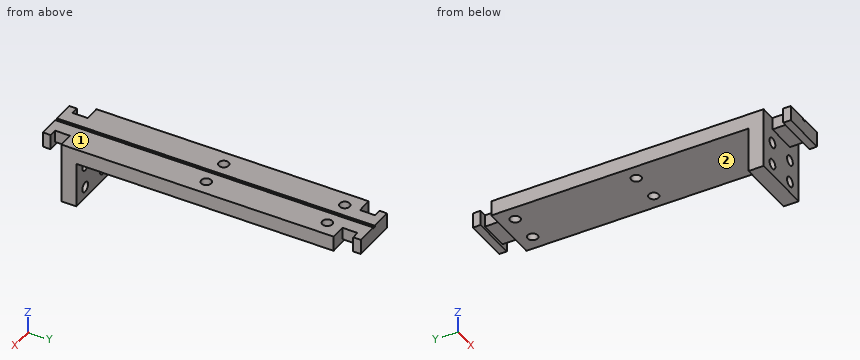
Autodesk Inventor part; units mm, degrees
ref_plane "YZ Plane" through (0, 0, 0) normal (1, 0, 0) x (0, 1, 0)
ref_plane "XZ Plane" through (0, 0, 0) normal (0, 1, 0) x (-1, 0, 0)
ref_plane "XY Plane" through (0, 0, 0) normal (0, 0, 1) x (1, 0, 0)
sketch "Sketch1" plane through (0, 0, 0) normal (0, 0, 1) x (1, 0, 0)
  line L0 (0, 0) -> (20, 0)
  line L1 (20, 0) -> (20, -2.7984)
  line L2 (0, -2.7984) -> (0, 0)
  line L3 (0, 0) -> (20, 0)
  line L4 (20, 0) -> (20, -50)
  line L5 (20, -50) -> (0, -50)
  line L6 (0, -50) -> (0, 0)
  line L7 (0, 0) -> (5, 0)
  line L8 (0, -5) -> (0, 0)
  circle A0 centre (5, -5) radius 1.651
  line L9 (20, 0) -> (15, 0)
  line L10 (15, -5) -> (20, -5)
  line L11 (20, -5) -> (20, 0)
  circle A1 centre (15, -5) radius 1.651
  dimension "d1" = 20
  dimension "d2" = 50
  dimension "d6" = 5
  dimension "d7" = 5
  dimension "d9" = 3.302
extrude "Extrusion1" add sketch "Sketch1" along normal blind 5
sketch "Sketch2" plane through (0, 0, 5) normal (0, 0, 1) x (1, 0, 0)
  line L0 (20, 0) -> (0, 0)
  line L1 (10, 0) -> (5, 0)
  line L2 (5, 0) -> (5, 5)
  line L3 (5, 5) -> (10, 5)
  line L4 (10, 5) -> (10, 0)
  line L5 (10, 5) -> (2.5, 5)
  line L6 (2.5, 5) -> (2.5, 7.5)
  line L7 (2.5, 7.5) -> (10, 7.5)
  line L8 (10, 7.5) -> (10, 5)
  line L9 (2.5, 7.5) -> (17.5, 7.5)
  line L10 (17.5, 7.5) -> (17.5, 5)
  line L11 (17.5, 5) -> (2.5, 5)
  line L12 (2.5, 5) -> (2.5, 7.5)
  line L13 (10, 5) -> (15, 5)
  line L14 (15, 5) -> (15, 0)
  line L15 (15, 0) -> (10, 0)
  line L16 (10, 0) -> (10, 5)
  dimension "d12" = 5
  dimension "d13" = 5
  dimension "d14" = 7.5
  dimension "d15" = 2.5
  dimension "d16" = 15
  dimension "d17" = 2.5
  dimension "d18" = 5
  dimension "d19" = 5
extrude "Extrusion2" add sketch "Sketch2" against normal blind 5
sketch "Sketch3" plane through (0, 0, 0) normal (0, 0, -1) x (-1, 0, 0)
  line L0 (-5, 0) -> (-5, 5)
  line L1 (-5, 0) -> (-15, 0)
  line L2 (-15, 0) -> (-15, 5)
  line L3 (-15, 5) -> (-5, 5)
  line L4 (-5, 5) -> (-5, 0)
  point P0 (0, 0)
extrude "Extrusion3" cut sketch "Sketch3" against normal blind 1
sketch "Sketch4" plane through (0, 0, 0) normal (0, 0, -1) x (-1, 0, 0)
  line L0 (-5, 0) -> (0, 0)
  line L1 (-20, -50) -> (0, -50)
  line L2 (0, 0) -> (-20, 0)
  line L3 (-20, 0) -> (-20, -50)
  line L4 (-20, -50) -> (0, -50)
  line L5 (0, -50) -> (0, 0)
  line L6 (0, -50) -> (-5, -50)
  line L7 (-5, -50) -> (-5, -30)
  line L8 (-5, -30) -> (0, -30)
  line L9 (0, -30) -> (0, -50)
  line L10 (0, -50) -> (0, 0)
  line L11 (0, -50) -> (-5, -50)
  line L12 (-5, -50) -> (-5, -30)
  line L13 (-5, -30) -> (0, -30)
  line L14 (0, -30) -> (0, -50)
  line L15 (0, -50) -> (-20, -50)
  line L16 (-20, -50) -> (-20, -45)
  line L17 (-20, -45) -> (0, -45)
  line L18 (0, -45) -> (0, -50)
  dimension "d28" = 5
  dimension "d29" = 20
  dimension "d30" = 5
  dimension "d31" = 20
  dimension "d32" = 20
  dimension "d33" = 5
extrude "Extrusion4" add sketch "Sketch4" along normal blind 15 contours L17 L7 L1 L3 | L5 L1 L7 L17
sketch "Sketch5" plane through (0, 0, 5) normal (0, 0, 1) x (1, 0, 0)
  line L0 (20, -50) -> (20, 0)
  line L1 (20, 0) -> (0, 0)
  line L2 (0, 0) -> (0, -50)
  line L3 (0, -50) -> (20, -50)
  line L4 (20, -50) -> (20, 0)
  line L5 (10, -50) -> (15, -50)
  line L6 (15, -50) -> (15, -55)
  line L7 (15, -55) -> (10, -55)
  line L8 (10, -55) -> (10, -50)
  line L9 (15, -55) -> (5, -55)
  line L10 (5, -55) -> (5, -50)
  line L11 (5, -50) -> (15, -50)
  line L12 (15, -50) -> (15, -55)
  line L13 (10, -55) -> (17.5, -55)
  line L14 (17.5, -55) -> (17.5, -57.5)
  line L15 (17.5, -57.5) -> (10, -57.5)
  line L16 (10, -57.5) -> (10, -55)
  line L17 (17.5, -57.5) -> (2.5, -57.5)
  line L18 (2.5, -57.5) -> (2.5, -55)
  line L19 (2.5, -55) -> (17.5, -55)
  line L20 (17.5, -55) -> (17.5, -57.5)
  dimension "d36" = 5
  dimension "d37" = 5
  dimension "d38" = 10
  dimension "d39" = 5
  dimension "d40" = 7.5
  dimension "d41" = 2.5
  dimension "d42" = 15
  dimension "d43" = 2.5
extrude "Extrusion5" add sketch "Sketch5" against normal blind 5 contours L6 L7 L8 L3 | L8 L9 L10 L3 | L13 L14 L15 L16 L7 | L16 L17 L18 L19 L9
sketch "Sketch6" plane through (0, 0, 0) normal (0, 0, -1) x (-1, 0, 0)
  line L0 (-5, -55) -> (-5, -50)
  line L1 (-15, -50) -> (-5, -50)
  line L2 (-5, -55) -> (-15, -55)
  line L3 (-15, -55) -> (-15, -50)
  line L4 (-15, -50) -> (-5, -50)
  line L5 (-5, -50) -> (-5, -55)
  point P0 (0, 0)
extrude "Extrusion6" cut sketch "Sketch6" against normal blind 1
sketch "Sketch8" plane through (0, -45, 0) normal (0, 1, 0) x (1, 0, 0)
  line L0 (0, 15) -> (20, 15)
  line L1 (0, 15) -> (20, 15)
  line L2 (20, 15) -> (20, 0)
  line L3 (20, 0) -> (0, 0)
  line L4 (0, 0) -> (0, 15)
  line L5 (0, 0) -> (0, 15)
  line L6 (0, 7.5) -> (20, 7.5)
  line L7 (20, 0) -> (20, 15)
  line L8 (20, 0) -> (0, 15)
  line L9 (20, 15) -> (0, 0)
  line L10 (10, 7.5) -> (10, 15)
  line L11 (10, 7.5) -> (10, 0)
  line L12 (10, 7.5) -> (0, 0)
  line L13 (10, 7.5) -> (20, 0)
  line L14 (10, 7.5) -> (0, 15)
  line L15 (10, 7.5) -> (20, 15)
  circle A0 centre (5, 3.75) radius 1.651
  circle A1 centre (15, 3.75) radius 1.651
  circle A2 centre (15, 11.25) radius 1.651
  circle A3 centre (5, 11.25) radius 1.651
  dimension "d48" = 3.302
  dimension "d49" = 3.302
  dimension "d50" = 3.302
  dimension "d51" = 3.302
extrude "Extrusion7" cut sketch "Sketch8" against normal blind 5 contours A3 L8 | L8 A3 | A2 L9 | L9 A2 | A1 L8 | L8 A1 | A0 L9 | L9 A0
sketch "Sketch9" plane through (0, 0, 0) normal (0, 0, -1) x (-1, 0, 0)
  circle A0 centre (-15, -5) radius 1.651
  line L0 (-15, -3.349) -> (-15, 35)
  line L1 (-16.651, -5) -> (-20, -5)
  line L2 (-20, -5) -> (-20, 40)
  line L3 (-20, 40) -> (-15, 40)
  line L4 (-15, 40) -> (-15, -3.349)
  line L5 (0, -45) -> (0, 0)
  line L6 (-20, 40) -> (0, 40)
  line L7 (0, 40) -> (0, -5)
  line L8 (-20, -5) -> (-20, 40)
  line L9 (-15, 35) -> (0, 35)
  line L10 (0, 35) -> (0, 40)
  line L11 (0, 40) -> (-15, 40)
  line L12 (-15, 40) -> (-15, 35)
  circle A1 centre (-5, -5) radius 1.651
  line L13 (-5, -5) -> (0, -5)
  line L14 (0, -5) -> (0, 35)
  line L15 (0, 35) -> (-5, 35)
  line L16 (-5, 35) -> (-5, -3.349)
  circle A2 centre (-15, 35) radius 1.651
  circle A3 centre (-5, 35) radius 1.651
  line L17 (-15, 40) -> (-5, 40)
  line L18 (-5, 40) -> (-5, 45)
  line L19 (-5, 45) -> (-15, 45)
  line L20 (-15, 45) -> (-15, 40)
  line L21 (-15, 45) -> (-17.5, 45)
  line L22 (-17.5, 45) -> (-17.5, 47.5)
  line L23 (-17.5, 47.5) -> (-15, 47.5)
  line L24 (-15, 47.5) -> (-15, 45)
  line L25 (-17.5, 47.5) -> (0, 47.5)
  line L26 (0, 47.5) -> (0, 45)
  line L27 (0, 45) -> (-17.5, 45)
  line L28 (-17.5, 45) -> (-17.5, 47.5)
  line L29 (-17.5, 47.5) -> (-2.5, 47.5)
  line L30 (-2.5, 47.5) -> (-2.5, 45)
  line L31 (-2.5, 45) -> (-17.5, 45)
  line L32 (-17.5, 45) -> (-17.5, 47.5)
  arc A4 (-13.349, -5) -> (-16.651, -5) centre (-15, -5) ccw
  arc A5 (-3.349, -5) -> (-6.651, -5) centre (-5, -5) ccw
  arc A6 (-13.349, -5) -> (-16.651, -5) centre (-15, -5) ccw
  arc A7 (-3.349, -5) -> (-6.651, -5) centre (-5, -5) ccw
  line L33 (0, -5) -> (-3.349, -5)
  line L34 (-6.651, -5) -> (-13.349, -5)
  line L35 (-16.651, -5) -> (-20, -5)
  dimension "d54" = 40
  dimension "d55" = 45
  dimension "d56" = 3.302
  dimension "d57" = 3.302
  dimension "d58" = 10
  dimension "d59" = 5
  dimension "d60" = 2.5
  dimension "d61" = 2.5
  dimension "d62" = 17.5
  dimension "d63" = 2.5
  dimension "d64" = 15
  dimension "d65" = 2.5
extrude "Extrusion8" add sketch "Sketch9" against normal blind 5 contours A0 L0 A2 L9 A3 L16 A1 L34 | A0 L1 L2 L3 L4 A2 L0 | A2 L4 L0 | L0 L9 A2 | L16 A3 L9 L7 L5 L13 A1 | L4 A2 L9 | L4 L6 L7 L9 A3 A2 | A3 L9 L16 | L16 L9 A3 | L20 L19 L18 L6 | A3 L9 | L24 L25 L30 L27 L19 | L21 L22 L23 L24
sketch "Sketch10" plane through (0, 0, 0) normal (0, 0, -1) x (-1, 0, 0)
  circle A0 centre (-15, -5) radius 1.651
  line L0 (-15, -5) -> (-15, 35)
  line L1 (-15, -5) -> (25, -5) construction
  line L2 (-15, 35) -> (-5, 35)
  circle A1 centre (-15, 35) radius 1.651
  circle A2 centre (-5, 35) radius 1.651
  point P0 (0, 0)
  dimension "d68" = 40
  dimension "d69" = 90
  dimension "d70" = 10
  dimension "d71" = 3.302
  dimension "d72" = 3.302
extrude "Extrusion9" cut sketch "Sketch10" against normal blind 5 contours A2 | A1 L2 L0 | L0 L2 A1
sketch "Sketch11" plane through (0, 0, 0) normal (0, 0, -1) x (-1, 0, 0)
  line L0 (-15, 45) -> (-17.5, 45)
  line L1 (-5, 40) -> (0, 40)
  line L2 (-15, 45) -> (-5, 45)
  line L3 (-5, 45) -> (-5, 40)
  line L4 (-5, 40) -> (-15, 40)
  line L5 (-15, 40) -> (-15, 45)
  point P0 (0, 0)
extrude "Extrusion10" cut sketch "Sketch11" against normal blind 1
sketch "Sketch13" plane through (2.5, -57.5, 5) normal (0, -1, 0) x (1, 0, 0)
  line L0 (0, 0) -> (15, 0)
  line L1 (7.5, 0) -> (8, 0)
  line L2 (8, 0) -> (8, -0.5)
  line L3 (8, -0.5) -> (7.5, -0.5)
  line L4 (7.5, -0.5) -> (7.5, 0)
  line L5 (8, -0.5) -> (7, -0.5)
  line L6 (7, -0.5) -> (7, 0)
  line L7 (7, 0) -> (8, 0)
  line L8 (8, 0) -> (8, -0.5)
  point P0 (-2.5, -5)
  dimension "d77" = 0.5
  dimension "d78" = 0.5
  dimension "d79" = 1
  dimension "d80" = 0.5
extrude "Extrusion11" cut sketch "Sketch13" against normal blind 500
properties part number "Attachment"
The model under review builds one solid part; all positions refer to its coordinate system, in mm. Face numbers are marked on the shaded views. A direction names the side the tool comes from. Give positions to 0.01 mm unless a question says otherwise; leave off trailing zeros. Order: outer loops, then holes, each group sorted by start corner. A loop starts at its lowest first (then second) coordinate and runs counter-clockwise, first axis right, second up. Notation, with made-up numbers: M 88,82.5 L 142,82.5 A19 ccw 142,99.5 Z; hole C -20,-25 d8. An arc over 180 degrees is marked long. Answer in a Markdown table with one row per item. Add a question column.
1. Add section B-B on z = -11.25. State the section outline as (x, y) points, plus the area to 3 significant figures.
2. Add section A-A on y = -5. State the section outline as (x, z) points.
3. Machinability: for the marked faces 1 and 2, which of the approach directions +Z, -Z, +X, -X, +Y, -Y give a long, thin tool a straight path to every point of the face, cutting with its end or side? Answer none if there is none.
4. Add section C-C on y = 23.5. State the section outline as (x, z) points.
5. For pin 1 Ø3 at (x, y) = (11.5, -56.5) entering from -Z; pin 2 Ø2 at (y, z) = (45.5, 2) entering from +X; pin 3 Ø2 at (y, z) = (-52, 4) entering from -X; pin 4 Ø2 at (x, y) = (15, -5) entering from +Z, all flat-tipped, find the tip position at first contact; note any pin that passes through.
6. To check wall thickness, follow line 1 along Z through (x, y) = (5, -46.65); line 2 along Y through (x, z) = (16.75, 0.25); line 3 along Y through (x, z) = (13.75, 4). State the ranges of each line that lie inside material, in increasing order.
The answers:
| question | item | result |
|---|---|---|
| 1 | outline | M 0,-50 L 3.35,-50 L 3.35,-45 L 0,-45 Z; M 6.65,-50 L 13.35,-50 L 13.35,-45 L 6.65,-45 Z; M 16.65,-50 L 20,-50 L 20,-45 L 16.65,-45 Z |
| 1 | area | 67.0 mm2 |
| 2 | outline | M 0,0 L 3.35,0 L 3.35,5 L 0,5 Z; M 6.65,0 L 13.35,0 L 13.35,5 L 10.5,5 L 10.5,4.5 L 9.5,4.5 L 9.5,5 L 6.65,5 Z; M 16.65,0 L 20,0 L 20,5 L 16.65,5 Z |
| 3 | face 1 | +Z, +X, -X, +Y, -Y |
| 3 | face 2 | -Z, +X, -X, +Y |
| 4 | outline | M 0,0 L 20,0 L 20,5 L 10.5,5 L 10.5,4.5 L 9.5,4.5 L 9.5,5 L 0,5 Z |
| 5 | pin 1 | z = 0 |
| 5 | pin 2 | x = 17.5 |
| 5 | pin 3 | x = 5 |
| 5 | pin 4 | through |
| 6 | line 1 | -15 to -12.9, -9.6 to -5.4, -2.1 to 5 |
| 6 | line 2 | -57.5 to -55, -50 to 40, 45 to 47.5 |
| 6 | line 3 | -57.5 to -6.08, -3.92 to 33.92, 36.08 to 47.5 |
